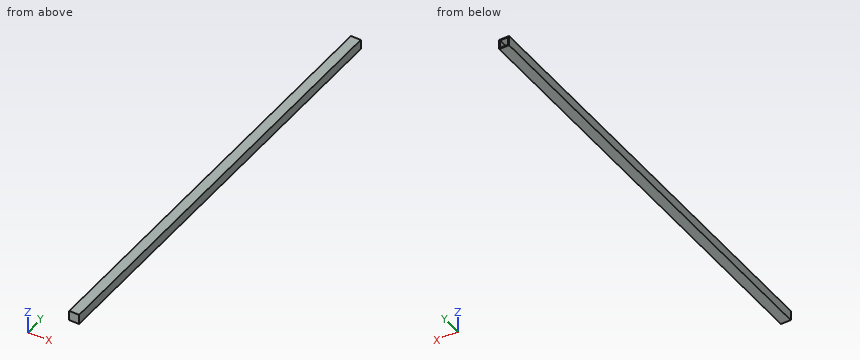
from build123d import *

# Parameters (mm, degrees)
SKETCH1_W           = 20
SKETCH1_H           = 900
BOSS_EXTRUDE1_DEPTH = 20
SKETCH2_W           = 16
SKETCH2_H           = 16
CUT_EXTRUDE1_DEPTH  = 200


with BuildPart() as part:
    # Sketch1 → Boss-Extrude1 (new body)
    with BuildSketch(Plane.XY):
        with Locations((-21.739130435, -400.217391304)):
            Rectangle(SKETCH1_W, SKETCH1_H)
    extrude(amount=-BOSS_EXTRUDE1_DEPTH)

    # Sketch2 → Cut-Extrude1 (cut)
    with BuildSketch(Plane(origin=(0, 49.782608696, 0), x_dir=(1, 0, 0), z_dir=(0, 1, 0))):
        with Locations((-21.739130435, 10)):
            Rectangle(SKETCH2_W, SKETCH2_H)
    extrude(amount=-CUT_EXTRUDE1_DEPTH, mode=Mode.SUBTRACT)


solid = part.part
Could you check a few things on this model? Use its own coordinates, in mm. Coordinates: 2 decimals unless noted, no trailing zeros. Order: outer loops, then holes, each group sorted by start corner. A loop starts at its lowest first (then second) coordinate and runs counter-clockwise, first axis right, second up.
Q1. Suppose I cut it at C-C on z = -7.5. Please give me the cut outline in (x, y).
Q2. Suppose I cut it at A-A on y = -31. Please give me the cut outline in (x, z).
Q3. Suppose I cut it at B-B on x = -18.5. Please give me the cut outline in (y, z), and give its area (3 significant figures).
Q4. Will this pin go through, and if not, where does the flat tip stop? pin 1 (5 mm diameter, centred on x = -21.5, z = -12, fed in from +Y).
Q5. Please list where these lines run through material, in increasing order: L1, parallel to X at y = 11.5, z = -10.5; L2, parallel to Z at x = -18, y = -16.5; L3, parallel to Y at x = -26.5, z = -16.75.
Answer:
1. outline: (-31.74, -850.22) - (-11.74, -850.22) - (-11.74, 49.78) - (-13.74, 49.78) - (-13.74, -150.22) - (-29.74, -150.22) - (-29.74, 49.78) - (-31.74, 49.78) - close
2. outline: (-31.74, -20) - (-11.74, -20) - (-11.74, 0) - (-31.74, 0) - close; hole (-29.74, -18) - (-13.74, -18) - (-13.74, -2) - (-29.74, -2) - close
3. outline: (-850.22, -20) - (49.78, -20) - (49.78, -18) - (-150.22, -18) - (-150.22, -2) - (49.78, -2) - (49.78, 0) - (-850.22, 0) - close
3. area: 14,800 mm2
4. pin 1: stops at y = -150.22
5. L1: x = -31.74 to -29.74, -13.74 to -11.74
5. L2: z = -20 to -18, -2 to 0
5. L3: y = -850.22 to -150.22
